Source: three-view drawing plus pictorial views. Frame: mm from the lowest corner of the part. A direction names the side the tool comes from. Coordinates: 2 decimals unless noted, no trailing zeros. Write each loop counter-clockwise with the first axis right and the second up, starting at its lowest first coordinate (ties: lowest second). Pieces come first, ordered by that corner, then holes. Notation, with made-up numbers: M -20.75,-21 L -7.75,-21 A20 ccw -7.75,12 Z; hole C 27,24 d5. An arc over 180 degrees is marked long. Write item = value, one per line. Start each with the question number.
Item 1: Pull-direction query (Z, two-part tool) for the marked faces 1, 2 and 3; classes: +Z half, -Z half, draft (parallel to the pull), parting line (faces both ways), or undercut.
Item 2: Reachability of the marked faces 4 and 5 from +Z, -Z, +X, -X, +Y, -Y: full face, straight path, thin tool, end or side. Return the list, or none.
Item 3: Section D-D on x = 64. Output: boundary loops of the cut face in (y, z).
Item 4: Section C-C on y = 81. Output: boundary loops of the cut face in (x, z), plus the area to 3 significant figures.
Item 5: Ray query, L1, parallel to X at y = 14.5, z = 65.5; L2, parallel to Z at x = 30, y = 53; L3, parallel to Z at x = 70, y = 67.5. Return the intervals inside material, ascending. Write a range as [from, to].
Item 6: First-contact query: pin 1 Ø12 at (x, z) = (27, 25.5) entering from +Y; pin 2 Ø3 at (x, z) = (79.5, 68) entering from -Y; pin 3 Ø8 at (x, y) = (59.5, 59) entering from +Z. Flat tips, straight axial feed; report the tip coordinate or a pass-through.
Item 7: Section A-A on y = 50.8. Output: boundary loops of the cut face in (x, z).
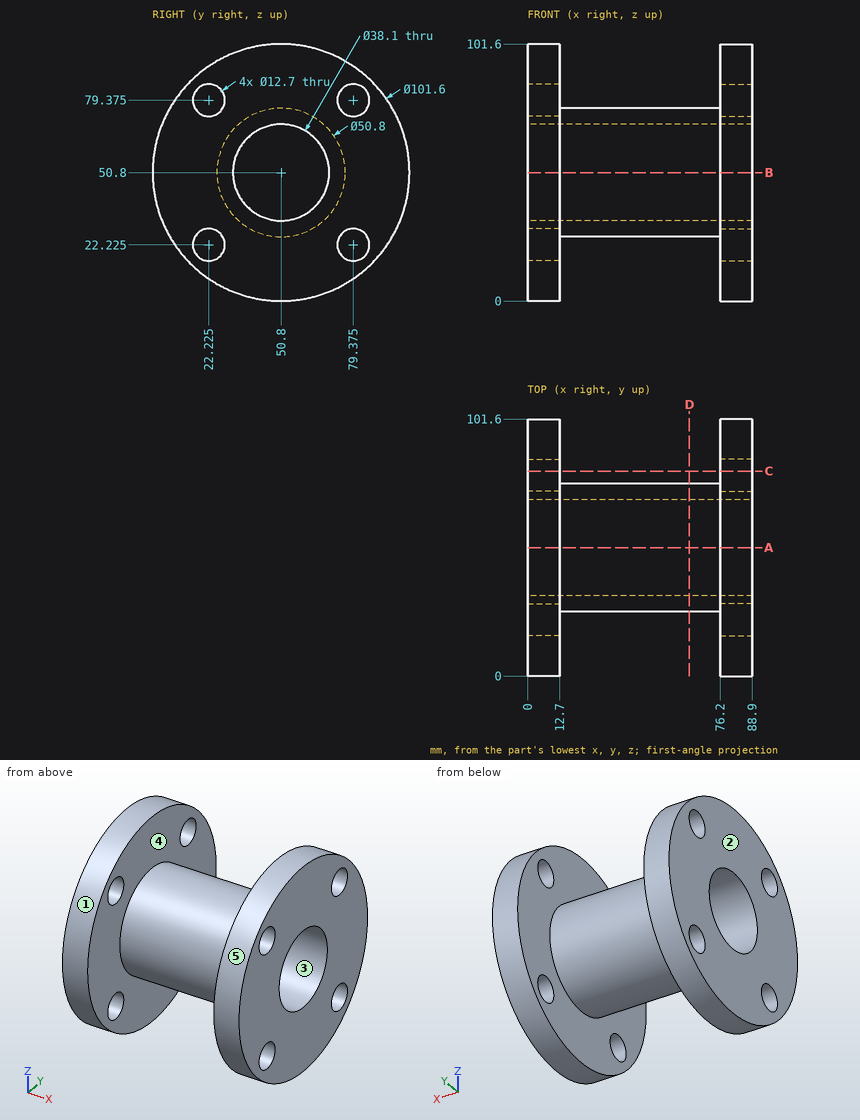
Responses:
q1.face_1 = parting line
q1.face_2 = draft
q1.face_3 = undercut
q2.face_4 = none
q2.face_5 = +X, -X
q3.outline = C 50.8,50.8 d50.8; hole C 50.8,50.8 d38.1
q4.outline = M 0,9.95 L 12.7,9.95 L 12.7,16.09 L 0,16.09 Z; M 0,28.36 L 12.7,28.36 L 12.7,73.24 L 0,73.24 Z; M 0,85.51 L 12.7,85.51 L 12.7,91.65 L 0,91.65 Z; M 76.2,9.95 L 88.9,9.95 L 88.9,16.09 L 76.2,16.09 Z; M 76.2,28.36 L 88.9,28.36 L 88.9,73.24 L 76.2,73.24 Z; M 76.2,85.51 L 88.9,85.51 L 88.9,91.65 L 76.2,91.65 Z
q4.area = 1,450 mm²
q5.L1 = [0, 12.7], [76.2, 88.9]
q5.L2 = [25.5, 31.88], [69.72, 76.1]
q5.L3 = [31.66, 41.63], [59.97, 69.94]
q6.pin_1 = 67.31
q6.pin_2 = 2.49
q6.pin_3 = 75.85
q7.outline = M 0,0 L 12.7,0 L 12.7,25.4 L 76.2,25.4 L 76.2,0 L 88.9,0 L 88.9,31.75 L 0,31.75 Z; M 0,69.85 L 88.9,69.85 L 88.9,101.6 L 76.2,101.6 L 76.2,76.2 L 12.7,76.2 L 12.7,101.6 L 0,101.6 Z
